Check sheet for the modelled part. Datum: model origin and axes. Units: mm. Face numbers are marked on the shaded views. A direction names the side the tool comes from. Give positions to 0.01 mm unless a question says otherwise; leave off trailing zeros. Order: outer loops, then holes, each group sorted by start corner. A loop starts at its lowest first (then second) coordinate and runs counter-clockwise, first axis right, second up.
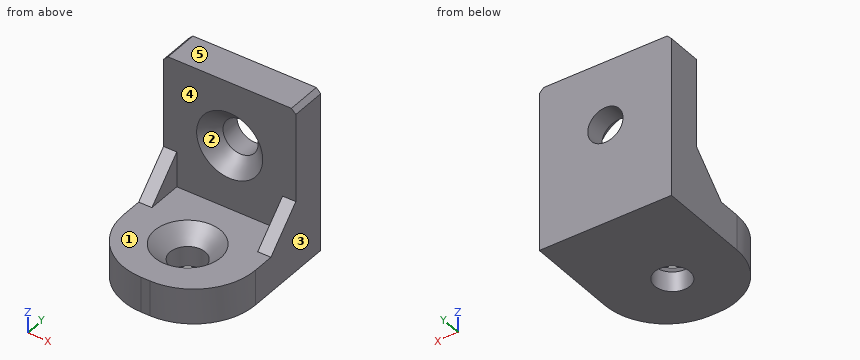
```python
from build123d import *

# Parameters (mm, degrees)
SKETCH_W        = 30
SKETCH_H        = 37
PAD_DEPTH       = 35
FILLET_R        = 14
BOX_W           = 32
BOX_H           = 32
BOX_DEPTH       = 32
SKETCH001_R     = 4
POCKET_DEPTH    = 8
SKETCH002_R     = 4
POCKET001_DEPTH = 8
CHAMFER_SIZE    = 3.5
CHAMFER001_SIZE = 1
SKETCH003_W     = 3
SKETCH003_H     = 8
PAD001_DEPTH    = 8
POCKET002_DEPTH = 30.001


with BuildPart() as part:
    # Sketch → Pad (new body)
    with BuildSketch(Plane.XZ):
        with Locations((0, 18.5)):
            Rectangle(SKETCH_W, SKETCH_H)
    extrude(amount=PAD_DEPTH)

    # Fillet
    fillet_edges = [part.edges().sort_by_distance(p)[0] for p in [
        (15, -35, 18.5),
        (-15, -35, 18.5),
    ]]
    fillet(fillet_edges, radius=FILLET_R)

    # Box → Box (cut)
    with BuildSketch(Plane(origin=(-16, -8, 8), x_dir=(1, 0, 0), z_dir=(0, -1, 0))):
        with Locations((16, 16)):
            Rectangle(BOX_W, BOX_H)
    extrude(amount=BOX_DEPTH, mode=Mode.SUBTRACT)

    # Sketch001 (on Face6 of Box) → Pocket (cut)
    with BuildSketch(Plane(origin=(0, -8, 22.5), x_dir=(1, 0, 0), z_dir=(0, -1, 0))):
        Circle(SKETCH001_R)
    extrude(amount=-POCKET_DEPTH, mode=Mode.SUBTRACT)

    # Sketch002 (on Face5 of Pocket) → Pocket001 (cut)
    with BuildSketch(Plane(origin=(0, -21.5, 8), x_dir=(-1, 0, 0), z_dir=(0, 0, 1))):
        Circle(SKETCH002_R)
    extrude(amount=-POCKET001_DEPTH, mode=Mode.SUBTRACT)

    # Chamfer
    chamfer_edges = [part.edges().sort_by_distance(p)[0] for p in [
        (-4, -8, 22.5),
        (4, -21.5, 8),
    ]]
    chamfer(chamfer_edges, length=CHAMFER_SIZE)

    # Chamfer001
    chamfer001_edges = [part.edges().sort_by_distance(p)[0] for p in [
        (15, -4, 37),
        (-15, -4, 37),
    ]]
    chamfer(chamfer001_edges, length=CHAMFER001_SIZE)

    # Sketch003 (on Face1 of Chamfer001) → Pad001 (join)
    with BuildSketch(Plane(origin=(0, -8, 8), x_dir=(1, 0, 0), z_dir=(0, -1, 0))):
        with Locations((13.5, 4)):
            Rectangle(SKETCH003_W, SKETCH003_H)
        with Locations((-13.5, 4)):
            Rectangle(SKETCH003_W, SKETCH003_H)
    extrude(amount=PAD001_DEPTH)

    # Sketch004 (on Face21 of Pad001) → Pocket002 (cut, through all)
    with BuildSketch(Plane(origin=(15, -8, 8), x_dir=(0, 0, 1), z_dir=(1, 0, 0))):
        Polygon((0, 8), (8, 0), (8, 8), align=None)
    extrude(amount=-POCKET002_DEPTH, mode=Mode.SUBTRACT)


solid = part.part
```
Q1. Tool access check on the marked faces 1 and 2. Record the directions out of +Z, -Z, +X, -X, +Y, -Y that give a thin tool (end or side, any length) a straight path to the whole face; none if there is none.
Q2. Sectioned sample at A-A, the plane z = 4. Record the cut outline in (x, y).
Q3. Sectioned sample at C-C, the plane x = 0. Record the cut outline in (y, z).
Q4. Sectioned sample at D-D, the plane y = -21.5. Record the cut outline in (x, z).
Q5. Go/stop test with flat-tipped pins: P1, Ø2, axis at x = -0.5, y = -15.5, coming from the +Z side; P2, Ø2, axis at x = -11.5, z = 19.5, coming from the +Y side; P3, Ø6.5, axis at x = 0, z = 22.5, coming from the +Y side; P4, Ø9, axis at x = 0, y = -21.5, coming from the +Z side. Record where each tip stops, or that it passes through.
Q6. Material ranges on line 1 (Z direction, x = 0, y = -2.55); line 2 (X direction, y = -21.5, z = 1.2); line 3 (Y direction, x = 0, z = 1.8), recorded low to high.
Q7. Sectioned sample at B-B, the plane z = 22.5. Record the cut outline in (x, y), plus the area to 3 significant figures.
Q8. Draft check along X on the marked faces 3, 4 and 5. Enter one of: pulls with the +X half, pulls with the -X half, needs draft (parallel to the pull), parting line crosses it, or undercut.
Filled in:
1. face 1: +Z, -Y
1. face 2: -Y
2. outline: (-15, -21) arc R14 ccw to (-1, -35) - (1, -35) arc R14 ccw to (15, -21) - (15, 0) - (-15, 0) - close; hole circle Ø8 at (0, -21.5)
3. outline: (-35, 0) - (-25.5, 0) - (-25.5, 4.5) - (-29, 8) - (-35, 8) - close; (-17.5, 0) - (0, 0) - (0, 18.5) - (-4.5, 18.5) - (-8, 15) - (-8, 8) - (-14, 8) - (-17.5, 4.5) - close; (-8, 30) - (-4.5, 26.5) - (0, 26.5) - (0, 37) - (-8, 37) - close
4. outline: (-14.99, 0) - (-4, 0) - (-4, 4.5) - (-7.5, 8) - (-14.99, 8) - close; (4, 0) - (14.99, 0) - (14.99, 8) - (7.5, 8) - (4, 4.5) - close
5. P1: stops at z = 7.52
5. P2: stops at y = 0
5. P3: passes through
5. P4: stops at z = 5
6. line 1: z = 0 to 18.5, 26.5 to 37
6. line 2: x = -14.99 to -4, 4 to 14.99
6. line 3: y = -35 to -25.5, -17.5 to 0
7. outline: (-15, -8) - (-7.5, -8) - (-4, -4.5) - (-4, 0) - (-15, 0) - close; (4, -4.5) - (7.5, -8) - (15, -8) - (15, 0) - (4, 0) - close
7. area: 164 mm2
8. face 3: pulls with the +X half
8. face 4: undercut
8. face 5: needs draft
